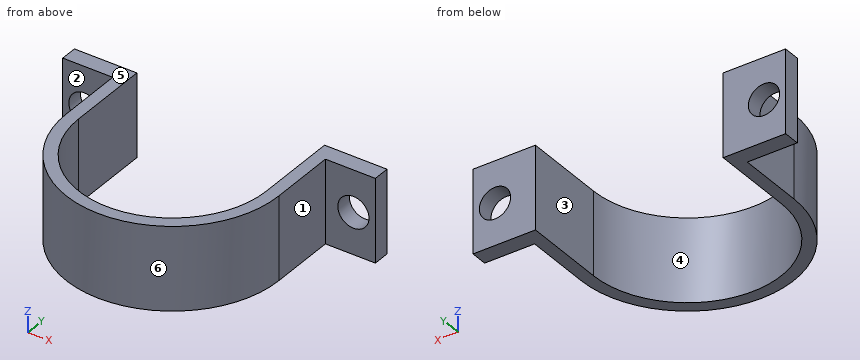
from build123d import *

# Parameters (mm, degrees)
BOSS_EXTRUDE2_DEPTH = 25.4
SKETCH5_R           = 4.7625
CUT_EXTRUDE1_DEPTH  = 38.1


with BuildPart() as part:
    # Sketch4 → Boss-Extrude2 (new body)
    with BuildSketch(Plane.XY):
        with BuildLine():
            Line((-32.385, 15.24), (-47.625, 15.24))
            Line((-47.625, 15.24), (-47.625, 20.32))
            Line((-47.625, 20.32), (-28.575, 20.32))
            Line((-28.575, 20.32), (-28.575, -5.08))
            ThreePointArc((-28.575, -5.08), (0.048187712, -33.703187712), (28.671375425, -5.08))
            Line((28.671375425, -5.08), (28.671375425, 20.32))
            Line((28.671375425, 20.32), (47.721375425, 20.32))
            Line((47.721375425, 20.32), (47.721375425, 15.24))
            Line((47.721375425, 15.24), (32.481375425, 15.24))
            Line((32.481375425, 15.24), (32.481375425, -5.08))
            ThreePointArc((32.481375425, -5.08), (0.048187712, -37.513187712), (-32.385, -5.08))
            Line((-32.385, -5.08), (-32.385, 15.24))
        make_face()
    extrude(amount=BOSS_EXTRUDE2_DEPTH)

    # Sketch5 → Cut-Extrude1 (cut)
    with BuildSketch(Plane(origin=(0, 20.32, 0), x_dir=(1, 0, 0), z_dir=(0, 1, 0))):
        with Locations(Location((-41.021, -12.7, 0), (0, 0, 180))):
            Circle(SKETCH5_R)
        with Locations(Location((41.021, -12.7, 0), (0, 0, 180))):
            Circle(SKETCH5_R)
    extrude(amount=-CUT_EXTRUDE1_DEPTH, mode=Mode.SUBTRACT)


solid = part.part
Geometry check sheet. Reference: the model listing, model coordinates, mm. Face numbers are marked on the shaded views. A direction names the side the tool comes from. Round coordinates to 2 decimals unless told otherwise and drop trailing zeros. Order: outer loops, then holes, each group sorted by start corner. A loop starts at its lowest first (then second) coordinate and runs counter-clockwise, first axis right, second up. Notation, with made-up numbers: M 85,-17 L 103,-17 A14 ccw 103,0 Z; hole C -0.5,24.5 d10. An arc over 180 degrees is marked long. Answer in a Markdown table with one row per item.
(1) Sectioned sample at C-C, the plane z = 5. Record the cut outline in (x, y) (3 decimals).
Responses:
| item | result |
|---|---|
| outline | M -47.625,15.24 L -32.385,15.24 L -32.385,-5.08 A32.433 ccw 32.481,-5.08 L 32.481,15.24 L 47.721,15.24 L 47.721,20.32 L 28.671,20.32 L 28.671,-5.08 A28.623 cw -28.575,-5.08 L -28.575,20.32 L -47.625,20.32 Z |
(2) Draft check along X on the marked faces 4, 5 and 6. Enter one of: released by +X, released by -X, zero draft, split by the parting line, or undercut.
Responses:
| item | result |
|---|---|
| face 4 | undercut |
| face 5 | zero draft |
| face 6 | split by the parting line |
(3) Sectioned sample at D-D, the plane y = -8. Record the cut outline in (x, z), and give its area (3 significant figures).
Responses:
| item | result |
|---|---|
| outline | M -32.25,0 L -28.43,0 L -28.43,25.4 L -32.25,25.4 Z; M 28.52,0 L 32.35,0 L 32.35,25.4 L 28.52,25.4 Z |
| area | 194 mm² |
(4) Sectioned sample at B-B, the plane y = -1.5. Record the cut outline in (x, z) (3 decimals).
Responses:
| item | result |
|---|---|
| outline | M -32.385,0 L -28.575,0 L -28.575,25.4 L -32.385,25.4 Z; M 28.671,0 L 32.481,0 L 32.481,25.4 L 28.671,25.4 Z |
(5) Tool access check on the marked faces 1, 2 and 3. Record the directions out of +Z, -Z, +X, -X, +Y, -Y that give a thin tool (end or side, any length) a straight path to the whole face; none if there is none.
Responses:
| item | result |
|---|---|
| face 1 | +Z, -Z, +X, -Y |
| face 2 | +Z, -Z, -X, -Y |
| face 3 | +Z, -Z, +Y |
(6) Sectioned sample at A-A, the plane z = 12.7. Record the cut outline in (x, y) (1 decimal).
Responses:
| item | result |
|---|---|
| outline | M -47.6,15.2 L -45.8,15.2 L -45.8,20.3 L -47.6,20.3 Z; M -36.3,15.2 L -32.4,15.2 L -32.4,-5.1 A32.4 ccw 32.5,-5.1 L 32.5,15.2 L 36.3,15.2 L 36.3,20.3 L 28.7,20.3 L 28.7,-5.1 A28.6 cw -28.6,-5.1 L -28.6,20.3 L -36.3,20.3 Z; M 45.8,15.2 L 47.7,15.2 L 47.7,20.3 L 45.8,20.3 Z |
(7) Go/stop test with flat-tipped pins: P1, Ø3, axis at y = 9.5, z = 4, coming from the +X side; P2, Ø10, axis at y = -16, z = 14, coming from the +X side; P3, Ø12, axis at x = -24, z = 20, coming from the -Y side. Record where each tip stops, or that it passes through.
Responses:
| item | result |
|---|---|
| P1 | stops at x = 32.48 |
| P2 | stops at x = 31.94 |
| P3 | stops at y = -32.03 |
(8) Scan lines: probe 1 along X at (y, z) = (11, 7) (3 decimals); probe 2 along X at (y, z) = (-24.5, 18); probe 3 along Y at (x, z) = (-40.5, 22). Record each from-to range of solid material in increasing order. Write a range as from..to.
Responses:
| item | result |
|---|---|
| probe 1 | x = -32.385..-28.575, 28.671..32.481 |
| probe 2 | x = -25.93..-20.98, 21.08..26.02 |
| probe 3 | y = 15.24..20.32 |
